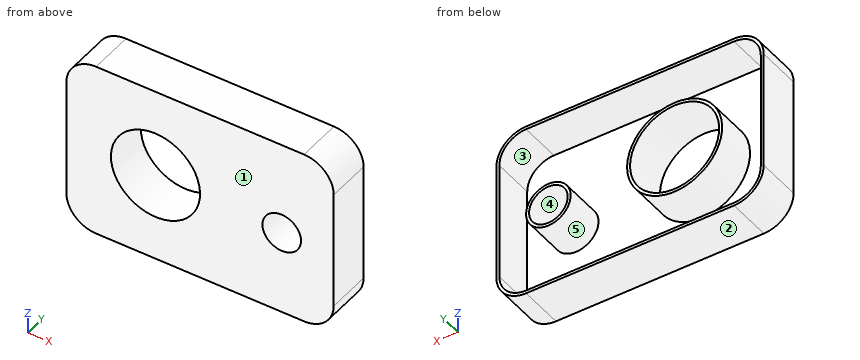
from build123d import *

# Parameters (mm, degrees)
SKETCH1_W           = 180
SKETCH1_H           = 120
BOSS_EXTRUDE1_DEPTH = 30
SKETCH4_R           = 30
SKETCH4_R_2         = 13
CUT_EXTRUDE1_DEPTH  = 219.403296678
FILLET1_R           = 20
SHELL2_T            = -2


with BuildPart() as part:
    # Sketch1 → Boss-Extrude1 (new body)
    with BuildSketch(Plane(origin=(0, 0, 0), x_dir=(1, 0, 0), z_dir=(0, 1, 0))):
        with Locations((90, -60)):
            Rectangle(SKETCH1_W, SKETCH1_H)
    extrude(amount=BOSS_EXTRUDE1_DEPTH)

    # Sketch4 → Cut-Extrude1 (cut, through all)
    with BuildSketch(Plane(origin=(0, 30, 0), x_dir=(1, 0, 0), z_dir=(0, 1, 0))):
        with Locations(Location((60, -60, 0), (0, 0, 270))):
            Circle(SKETCH4_R)
        with Locations(Location((145, -56.926363362, 0), (0, 0, 270))):
            Circle(SKETCH4_R_2)
    extrude(amount=-CUT_EXTRUDE1_DEPTH, mode=Mode.SUBTRACT)

    # Fillet1
    fillet1_edges = [part.edges().sort_by_distance(p)[0] for p in [
        (0, 15, 0),
        (180, 15, 0),
        (180, 15, 120),
        (0, 15, 120),
    ]]
    fillet(fillet1_edges, radius=FILLET1_R)

    # Shell2
    shell2_openings = [part.faces().sort_by_distance(p)[0] for p in [
        (93.107668166, 30, 60.091175454),
    ]]
    offset(amount=SHELL2_T, openings=shell2_openings, kind=Kind.INTERSECTION)


solid = part.part
Geometry check sheet. Reference: the model listing, model coordinates, mm. Face numbers are marked on the shaded views. A direction names the side the tool comes from. Round coordinates to 2 decimals unless told otherwise and drop trailing zeros. Loops run counter-clockwise (first coordinate to the right, second up) from the corner with the lowest first, then second, coordinate; pieces in that order, holes last.
Item 1: Gauge pin test, flat ends, axial feed: pin 1 (4 mm diameter, centred on y = 10.5, z = 15.5, fed in from -X); pin 2 (12 mm diameter, centred on x = 47.5, z = 99.5, fed in from +Y); pin 3 (4 mm diameter, centred on y = 7.5, z = 15, fed in from +X). Record the tip position at first contact, or that the pin passes through.
Item 2: Cross-section at C-C on z = 84.5. Record the boundary of the cut face in (x, y).
Item 3: Mould release check, pull along Z, two halves, no side actions. Record for the marked faces 1, 2 and 3: pulls with the +Z half, pulls with the -Z half, needs draft (parallel to the pull), parting line crosses it, or undercut.
Item 4: Thickness scan on line 1 (Z direction, x = 144, y = 12.5); line 2 (Z direction, x = 120.5, y = 16); line 3 (Z direction, x = 63, y = 11.25). Record the ranges inside material, lowest first.
Item 5: Cross-section at B-B on y = 18.25. Record the boundary of the cut face in (x, z), then the cut area to 3 significant figures.
Item 6: Access from +Z, -Z, +X, -X, +Y, -Y to the whole of each face (thin tool, end or side, straight path). Record for the marked faces 4 and 5.
Item 7: Cross-section at D-D on z = 49. Record the boundary of the cut face in (x, y), then the cut area to 3 significant figures.
Item 8: Cross-section at A-A on x = 145. Record the boundary of the cut face in (y, z).
Answer sheet:
1. pin 1: stops at x = 0.16
1. pin 2: stops at y = 2
1. pin 3: stops at x = 179.77
2. outline: (0, 0) - (42.69, 0) - (42.69, 30) - (39.41, 30) - (39.41, 2) - (2, 2) - (2, 30) - (0, 30) - close; (77.31, 0) - (180, 0) - (180, 30) - (178, 30) - (178, 2) - (80.59, 2) - (80.59, 30) - (77.31, 30) - close
3. face 1: needs draft
3. face 2: pulls with the -Z half
3. face 3: undercut
4. line 1: z = 0 to 2, 41.96 to 43.96, 69.89 to 71.89, 118 to 120
4. line 2: z = 0 to 2, 118 to 120
4. line 3: z = 0 to 2, 28.14 to 30.15, 89.85 to 91.86, 118 to 120
5. outline: (0, 20) arc R20 ccw to (20, 0) - (160, 0) arc R20 ccw to (180, 20) - (180, 100) arc R20 ccw to (160, 120) - (20, 120) arc R20 ccw to (0, 100) - close; circle Ø64 at (60, 60); circle Ø30 at (145, 56.93); hole (2, 20) arc R18 ccw to (20, 2) - (160, 2) arc R18 ccw to (178, 20) - (178, 100) arc R18 ccw to (160, 118) - (20, 118) arc R18 ccw to (2, 100) - close; hole circle Ø60 at (60, 60); hole circle Ø26 at (145, 56.93)
5. area: 1,680 mm2
6. face 4: +Y, -Y
6. face 5: +Y
7. outline: (0, 0) - (32.09, 0) - (32.09, 30) - (29.95, 30) - (29.95, 2) - (2, 2) - (2, 30) - (0, 30) - close; (87.91, 0) - (134.7, 0) - (134.7, 30) - (132.27, 30) - (132.27, 2) - (90.05, 2) - (90.05, 30) - (87.91, 30) - close; (155.3, 0) - (180, 0) - (180, 30) - (178, 30) - (178, 2) - (157.73, 2) - (157.73, 30) - (155.3, 30) - close
7. area: 575 mm2
8. outline: (0, 0) - (30, 0) - (30, 2) - (2, 2) - (2, 41.93) - (30, 41.93) - (30, 43.93) - (0, 43.93) - close; (0, 69.93) - (30, 69.93) - (30, 71.93) - (2, 71.93) - (2, 118) - (30, 118) - (30, 120) - (0, 120) - close
